CAD build for the part. Positions are in the model's coordinates, mm. A direction names the side the tool comes from. Give positions to 0.01 mm unless a question says otherwise; leave off trailing zeros. One line per question, with ' | ' between items.
Autodesk Inventor part; units mm, degrees
ref_plane "YZ Plane" through (0, 0, 0) normal (1, 0, 0) x (0, 1, 0)
ref_plane "XZ Plane" through (0, 0, 0) normal (0, 1, 0) x (-1, 0, 0)
ref_plane "XY Plane" through (0, 0, 0) normal (0, 0, 1) x (1, 0, 0)
sketch "Sketch1" plane through (0, 0, 0) normal (0, 0, 1) x (1, 0, 0)
  arc A0 (32.8389, -3.2565) -> (32.9574, -1.6756) centre (0, 0) ccw
  circle A1 centre (0, 0) radius 26.25
  line L0 (0, 0) -> (42.2346, 0) construction
  line L1 (0, 0) -> (37.3319, 0) construction
  arc A2 (32.9574, -1.6756) -> (26.2428, 0.6158) centre (26.4907, -9.6418) ccw
  line L2 (0, 0) -> (41.4252, 0) construction
  arc A3 (25.8577, -4.5212) -> (32.8389, -3.2565) centre (27.632, 5.5848) ccw
  arc A4 (32.238, 7.0507) -> (31.8622, 8.5908) centre (0, 0) ccw
  arc A5 (31.8622, 8.5908) -> (24.7681, 8.6951) centre (28.1736, -0.9838) ccw
  arc A6 (25.9893, 3.6905) -> (32.238, 7.0507) centre (24.5538, 13.8502) ccw
  arc A7 (28.4814, 16.6677) -> (27.648, 18.0163) centre (0, 0) ccw
  arc A8 (27.648, 18.0163) -> (20.8689, 15.9233) centre (27.0987, 7.7704) ccw
  arc A9 (23.5768, 11.541) -> (28.4814, 16.6677) centre (19.0721, 20.7599) ccw
  arc A10 (21.9368, 24.6531) -> (20.7275, 25.6782) centre (0, 0) ccw
  arc A11 (20.7275, 25.6782) -> (14.9269, 21.5928) centre (23.3712, 15.7641) ccw
  arc A12 (18.8565, 18.2618) -> (21.9368, 24.6531) centre (11.7235, 25.6375) ccw
  arc A13 (13.2449, 30.2254) -> (11.778, 30.8266) centre (0, 0) ccw
  arc A14 (11.778, 30.8266) -> (7.5238, 25.1487) centre (17.356, 22.2146) ccw
  arc A15 (12.2904, 23.195) -> (13.2449, 30.2254) centre (3.2273, 28.0054) ccw
  arc A16 (3.2565, 32.8389) -> (1.6756, 32.9574) centre (0, 0) ccw
  arc A17 (1.6756, 32.9574) -> (-0.6158, 26.2428) centre (9.6418, 26.4907) ccw
  arc A18 (4.5212, 25.8577) -> (3.2565, 32.8389) centre (-5.5848, 27.632) ccw
  arc A19 (-7.0507, 32.238) -> (-8.5908, 31.8622) centre (0, 0) ccw
  arc A20 (-8.5908, 31.8622) -> (-8.6951, 24.7681) centre (0.9838, 28.1736) ccw
  arc A21 (-3.6905, 25.9893) -> (-7.0507, 32.238) centre (-13.8502, 24.5538) ccw
  arc A22 (-16.6677, 28.4814) -> (-18.0163, 27.648) centre (0, 0) ccw
  arc A23 (-18.0163, 27.648) -> (-15.9233, 20.8689) centre (-7.7704, 27.0987) ccw
  arc A24 (-11.541, 23.5768) -> (-16.6677, 28.4814) centre (-20.7599, 19.0721) ccw
  arc A25 (-24.6531, 21.9368) -> (-25.6782, 20.7275) centre (0, 0) ccw
  arc A26 (-25.6782, 20.7275) -> (-21.5928, 14.9269) centre (-15.7641, 23.3712) ccw
  arc A27 (-18.2618, 18.8565) -> (-24.6531, 21.9368) centre (-25.6375, 11.7235) ccw
  arc A28 (-30.2254, 13.2449) -> (-30.8266, 11.778) centre (0, 0) ccw
  arc A29 (-30.8266, 11.778) -> (-25.1487, 7.5238) centre (-22.2146, 17.356) ccw
  arc A30 (-23.195, 12.2904) -> (-30.2254, 13.2449) centre (-28.0054, 3.2273) ccw
  arc A31 (-32.8389, 3.2565) -> (-32.9574, 1.6756) centre (0, 0) ccw
  arc A32 (-32.9574, 1.6756) -> (-26.2428, -0.6158) centre (-26.4907, 9.6418) ccw
  arc A33 (-25.8577, 4.5212) -> (-32.8389, 3.2565) centre (-27.632, -5.5848) ccw
  arc A34 (-32.238, -7.0507) -> (-31.8622, -8.5908) centre (0, 0) ccw
  arc A35 (-31.8622, -8.5908) -> (-24.7681, -8.6951) centre (-28.1736, 0.9838) ccw
  arc A36 (-25.9893, -3.6905) -> (-32.238, -7.0507) centre (-24.5538, -13.8502) ccw
  arc A37 (-28.4814, -16.6677) -> (-27.648, -18.0163) centre (0, 0) ccw
  arc A38 (-27.648, -18.0163) -> (-20.8689, -15.9233) centre (-27.0987, -7.7704) ccw
  arc A39 (-23.5768, -11.541) -> (-28.4814, -16.6677) centre (-19.0721, -20.7599) ccw
  arc A40 (-21.9368, -24.6531) -> (-20.7275, -25.6782) centre (0, 0) ccw
  arc A41 (-20.7275, -25.6782) -> (-14.9269, -21.5928) centre (-23.3712, -15.7641) ccw
  arc A42 (-18.8565, -18.2618) -> (-21.9368, -24.6531) centre (-11.7235, -25.6375) ccw
  arc A43 (-13.2449, -30.2254) -> (-11.778, -30.8266) centre (0, 0) ccw
  arc A44 (-11.778, -30.8266) -> (-7.5238, -25.1487) centre (-17.356, -22.2146) ccw
  arc A45 (-12.2904, -23.195) -> (-13.2449, -30.2254) centre (-3.2273, -28.0054) ccw
  arc A46 (-3.2565, -32.8389) -> (-1.6756, -32.9574) centre (0, 0) ccw
  arc A47 (-1.6756, -32.9574) -> (0.6158, -26.2428) centre (-9.6418, -26.4907) ccw
  arc A48 (-4.5212, -25.8577) -> (-3.2565, -32.8389) centre (5.5848, -27.632) ccw
  arc A49 (7.0507, -32.238) -> (8.5908, -31.8622) centre (0, 0) ccw
  arc A50 (8.5908, -31.8622) -> (8.6951, -24.7681) centre (-0.9838, -28.1736) ccw
  arc A51 (3.6905, -25.9893) -> (7.0507, -32.238) centre (13.8502, -24.5538) ccw
  arc A52 (16.6677, -28.4814) -> (18.0163, -27.648) centre (0, 0) ccw
  arc A53 (18.0163, -27.648) -> (15.9233, -20.8689) centre (7.7704, -27.0987) ccw
  arc A54 (11.541, -23.5768) -> (16.6677, -28.4814) centre (20.7599, -19.0721) ccw
  arc A55 (24.6531, -21.9368) -> (25.6782, -20.7275) centre (0, 0) ccw
  arc A56 (25.6782, -20.7275) -> (21.5928, -14.9269) centre (15.7641, -23.3712) ccw
  arc A57 (18.2618, -18.8565) -> (24.6531, -21.9368) centre (25.6375, -11.7235) ccw
  arc A58 (30.2254, -13.2449) -> (30.8266, -11.778) centre (0, 0) ccw
  arc A59 (30.8266, -11.778) -> (25.1487, -7.5238) centre (22.2146, -17.356) ccw
  arc A60 (23.195, -12.2904) -> (30.2254, -13.2449) centre (28.0054, -3.2273) ccw
  point P0 (35.5048, 11.5362)
  point P1 (30.2022, 21.9432)
  point P2 (21.9432, 30.2022)
  point P3 (11.5362, 35.5048)
  point P4 (0, 37.3319)
  point P5 (-11.5362, 35.5048)
  point P6 (-21.9432, 30.2022)
  point P7 (-30.2022, 21.9432)
  point P8 (-35.5048, 11.5362)
  point P9 (-37.3319, 0)
  point P10 (-35.5048, -11.5362)
  point P11 (-30.2022, -21.9432)
  point P12 (-21.9432, -30.2022)
  point P13 (-11.5362, -35.5048)
  point P14 (0, -37.3319)
  point P15 (11.5362, -35.5048)
  point P16 (21.9432, -30.2022)
  point P17 (30.2022, -21.9432)
  point P18 (35.5048, -11.5362)
  point P19 (-14.9269, -21.5928)
  point P20 (-12.2904, -23.195)
  point P21 (-7.5238, -25.1487)
  point P22 (0.6158, -26.2428)
  point P23 (3.6905, -25.9893)
  point P24 (18.2618, -18.8565)
  point P25 (21.5928, -14.9269)
  point P26 (23.195, -12.2904)
  point P27 (25.1487, -7.5238)
  point P28 (25.9893, 3.6905)
  point P29 (20.8689, 15.9233)
  point P30 (18.8565, 18.2618)
  point P31 (14.9269, 21.5928)
  point P32 (7.5238, 25.1487)
  point P33 (-0.6158, 26.2428)
  point P34 (-3.6905, 25.9893)
  point P35 (-15.9233, 20.8689)
  point P36 (-18.2618, 18.8565)
  point P37 (-21.5928, 14.9269)
  point P38 (-23.195, 12.2904)
  point P39 (-25.1487, 7.5238)
  point P40 (-26.2428, -0.6158)
  point P41 (-24.7681, -8.6951)
  point P42 (-20.8689, -15.9233)
  point P43 (-18.8565, -18.2618)
  dimension "d2" = 52.5
  dimension "d1" = 66
  dimension "d13" = 360
extrude "Extrusion1" add sketch "Sketch1" along normal blind 15
sketch "Sketch2" plane through (0, 0, 15) normal (0, 0, 1) x (1, 0, 0)
  circle A0 centre (0, 0) radius 2.5
  line L0 (0, 2.5) -> (0, -1.7)
  line L1 (0, -1.7) -> (-3.9911, -1.7)
  line L2 (-3.9911, -1.7) -> (4.1911, -1.7)
  point P0 (1.833, -1.7)
  point P1 (-1.833, -1.7)
  dimension "d17" = 5
  dimension "d22" = 4.2
extrude "Extrusion2" cut sketch "Sketch2" against normal blind 15 contours A0 L2 L0 | L0 L1 A0
properties part number "ENGRANE MOTRIZ DE CAJA"
Item 1: Drop flat-ended pins along their axis: P1, Ø2, axis at y = -18.5, z = 13, coming from the +X side; P2, Ø3, axis at x = -0.5, z = 5, coming from the +Y side; P3, Ø1, axis at y = 5, z = 12.5, coming from the +X side; P4, Ø4, axis at y = 0, z = 9, coming from the -X side. Give the stop position or say it passes through.
Conclusion:
P1: x = 25.27 | P2: y = 32.02 | P3: x = 30.52 | P4: x = -32.96
Item 2: Mould opens along X. For faces 5 (the cylindrical face through (28.326, -9.114, 7.395)), 6 (the cylindrical face through (-32.057, -7.834, 7.395)), 7 (the cylindrical face through (-28.274, -9.276, 7.395)) say: pulls with the +X half, pulls with the -X half, needs draft (parallel to the pull), parting line crosses it, or undercut.
Conclusion:
face 5: pulls with the +X half | face 6: pulls with the -X half | face 7: undercut
Item 3: 3-axis set-ups, long thin cutter, end or side, ignore diameter. For faces 1 (the cylindrical face through (26.52, 13.7, 7.4)), 2 (the cylindrical face through (-2.18, 26.16, 7.4)), 3 (the cylindrical face through (2.18, -26.16, 7.4)), 4 (the cylindrical face through (17.56, -24.02, 7.4)): which of +Z, -Z, +X, -X, +Y, -Y reach the whole face in a straight line?
Conclusion:
face 1: +Z, -Z, +X | face 2: +Z, -Z, +Y | face 3: +Z, -Z, -Y | face 4: +Z, -Z
Item 4: Drill centre lines: line 1 along Y through (x, z) = (19, 9.25); line 2 along X through (y, z) = (28, 11.5); line 3 along Y through (x, z) = (23.5, 4). Where is each one in solid material? Low to high. Write a range as [from, to].
Conclusion:
line 1: [-19.55, 18.11], [18.4, 25.05] | line 2: [-17.46, -15.7], [-9.28, -4.19], [-0.51, 4.67], [8.88, 13.49] | line 3: [-21.76, -16.63], [-12.45, 17.38]
